from build123d import *

# Parameters (mm, degrees)
SKETCH1_W           = 24.4
SKETCH1_H           = 33.5
BOSS_EXTRUDE1_DEPTH = 41.5
BOSS_EXTRUDE2_DEPTH = 3
SKETCH4_W           = 11
SKETCH4_H           = 1.5
BOSS_EXTRUDE3_DEPTH = 11.5
CUT_EXTRUDE1_DEPTH  = 25.4
FILLET1_R           = 2


with BuildPart() as part:
    # Sketch1 → Boss-Extrude1 (new body)
    with BuildSketch(Plane(origin=(0, 0, 0), x_dir=(1, 0, 0), z_dir=(0, 1, 0))):
        with Locations((12.2, 16.75)):
            Rectangle(SKETCH1_W, SKETCH1_H)
    extrude(amount=BOSS_EXTRUDE1_DEPTH)

    # Sketch3 → Boss-Extrude2 (add)
    with BuildSketch(Plane.XZ):
        Polygon((0, 0), (24.4, 0), (24.4, -14.5), (17.95, -14.5), (17.95, -27.5), (6.45, -27.5), (6.45, -14.5), (0, -14.5), align=None)
    extrude(amount=BOSS_EXTRUDE2_DEPTH)

    # Sketch4 → Boss-Extrude3 (add)
    with BuildSketch(Plane(origin=(0, 41.5, 0), x_dir=(-1, 0, 0), z_dir=(0, 1, 0))):
        with Locations((-5.5, -32.75)):
            Rectangle(SKETCH4_W, SKETCH4_H)
    extrude(amount=BOSS_EXTRUDE3_DEPTH)

    # Sketch5 → Cut-Extrude1 (cut, through all)
    with BuildSketch(Plane(origin=(24.4, 0, 0), x_dir=(0, 0, -1), z_dir=(1, 0, 0))):
        Polygon((33.5, 0), (31.46940795, 0), (31.797940048, 39.10064674), (33.5, 39.10064674), align=None)
    extrude(amount=-CUT_EXTRUDE1_DEPTH, mode=Mode.SUBTRACT)

    # Fillet1
    fillet1_edges = [part.edges().sort_by_distance(p)[0] for p in [
        (0, 53, -32.75),
        (11, 53, -32.75),
    ]]
    fillet(fillet1_edges, radius=FILLET1_R)


solid = part.part
Build history of the part. All positions in model axes, mm. A direction names the side the tool comes from. Give positions to 0.01 mm unless a question says otherwise; leave off trailing zeros. Loops run counter-clockwise (first coordinate to the right, second up) from the corner with the lowest first, then second, coordinate; pieces in that order, holes last. Notation, with made-up numbers: (16, -6) -> (59, -6) arc R12 ccw to (59, 12) -> close; hole circle Ø3 at (-34.5, 51). An arc over 180 degrees is marked (long way). Answer in a Markdown table with one row per item.
Item 1: Slice it at D-D on x = 3.5. Write the cut outline in (y, z).
Findings below:
| item | result |
|---|---|
| outline | (-3, -14.5) -> (0, -14.5) -> (0, -31.47) -> (39.1, -31.8) -> (39.1, -33.5) -> (53, -33.5) -> (53, -32) -> (41.5, -32) -> (41.5, 0) -> (-3, 0) -> close |
Item 2: Probe line 1 along Y through (x, z) = (7, -16); line 2 along Y through (x, z) = (2, -30); line 3 along Z through (x, y) = (21, 0.5). List the from-to ranges inside material, lowest first. Write a range as [from, to].
Findings below:
| item | result |
|---|---|
| line 1 | y = [-3, 41.5] |
| line 2 | y = [0, 41.5] |
| line 3 | z = [-31.47, 0] |
Item 3: Slice it at B-B on z = -26.5. Write the cut outline in (x, y).
Findings below:
| item | result |
|---|---|
| outline | (0, 0) -> (6.45, 0) -> (6.45, -3) -> (17.95, -3) -> (17.95, 0) -> (24.4, 0) -> (24.4, 41.5) -> (0, 41.5) -> close |
Item 4: Tool access for faces 1 (the flat face through (6, 47, -32)), 2 (the flat face through (12, 39.101, -33)), 3 (the flat face through (3, -1, -14.5)), 4 (the flat face through (21, -1, -14.5)): list every direction of +Z, -Z, +X, -X, +Y, -Y with a clear straight run to the whole face (end or side of a thin tool).
Findings below:
| item | result |
|---|---|
| face 1 | +Z, +X, -X, +Y |
| face 2 | -Z, +X, -X, -Y |
| face 3 | -Z, -X, -Y |
| face 4 | -Z, +X, -Y |
Item 5: Flat gauge pins, fed straight in: P1, Ø6, axis at x = 11, y = 23.5, coming from the +Z side; P2, Ø0.9, axis at x = 3.5, y = -1.5, coming from the -Z side; P3, Ø3.5, axis at x = 14.5, y = -1.5, coming from the -Z side; P4, Ø5, axis at x = 15, z = -19.5, coming from the +Y side. Where does each tip first touch, or does it go through?
Findings below:
| item | result |
|---|---|
| P1 | stops at z = 0 |
| P2 | stops at z = -14.5 |
| P3 | stops at z = -31.47 |
| P4 | stops at y = 41.5 |
Item 6: Slice it at A-A on x = 14.75. Write the cut outline in (y, z).
Findings below:
| item | result |
|---|---|
| outline | (-3, -27.5) -> (0, -27.5) -> (0, -31.47) -> (39.1, -31.8) -> (39.1, -33.5) -> (41.5, -33.5) -> (41.5, 0) -> (-3, 0) -> close |
Item 7: Slice it at C-C on y = 47. Write the cut outline in (x, z), plus the area to 3 significant figures.
Findings below:
| item | result |
|---|---|
| outline | (0, -33.5) -> (11, -33.5) -> (11, -32) -> (0, -32) -> close |
| area | 16.5 mm² |
